Work out the finished part from the listing and answer in its coordinate system (mm). A direction names the side the tool comes from. Coordinates: 2 decimals unless noted, no trailing zeros. Write each loop counter-clockwise with the first axis right and the second up, starting at its lowest first coordinate (ties: lowest second). Pieces come first, ordered by that corner, then holes. Notation, with made-up numbers: M -39,10 L 19,10 A7 cw 19,18 Z; hole C 14,11.25 d2. An arc over 180 degrees is marked long. Use CSV: the item, a comma, the result in double quotes.
from build123d import *

# Parameters (mm, degrees)
CUT_EXTRUDE1_DEPTH      = 126.267501457
CUT_EXTRUDE1_DEPTH_BACK = 126.267501457
SKETCH2_R               = 2.986936388
CUT_EXTRUDE2_DEPTH      = 126.267501556
CUT_EXTRUDE2_DEPTH_BACK = 126.267501556


with BuildPart() as part:
    # Sketch1 → Revolve1 (revolve)
    with BuildSketch(Plane(origin=(0, 0, 0), x_dir=(0, 0, -1), z_dir=(1, 0, 0)), mode=Mode.PRIVATE) as revolve1_sk:
        Polygon((0, 123.60144971), (12, 123.60144971), (12, 86.261621461), (14.398412253, 86.261621461), (14.398412253, 79.261621461), (6.991481123, 79.261621461), (6.991481123, 8.748152398), (13.363236745, 8.748152398), (13.363236745, 3.47746721), (0, 3.47746721), align=None)
    revolve(revolve1_sk.sketch.rotate(Axis((0, 123.60144971, 0), (0, -1, 0)), 180), axis=Axis((0, 123.60144971, 0), (0, -1, 0)))

    # Sketch2 → Cut-Extrude1 (cut, two sides: drawn at the far end of the back side and taken through both)
    with BuildSketch(Plane(origin=(0, 0, 0), x_dir=(0, 0, -1), z_dir=(1, 0, 0)).offset(-CUT_EXTRUDE1_DEPTH_BACK)):
        with Locations((0, 113.066011559)):
            Circle(SKETCH2_R)
    extrude(amount=CUT_EXTRUDE1_DEPTH + CUT_EXTRUDE1_DEPTH_BACK, mode=Mode.SUBTRACT)

    # Sketch3 → Cut-Extrude2 (cut, two sides: drawn at the far end of the back side and taken through both)
    with BuildSketch(Plane(origin=(0, 0, 0), x_dir=(0, 0, -1), z_dir=(1, 0, 0)).offset(-CUT_EXTRUDE2_DEPTH_BACK)):
        with BuildLine():
            Line((1.8, 55.325549997), (1.8, 35.81578841))
            ThreePointArc((1.8, 35.81578841), (0, 34.01578841), (-1.8, 35.81578841))
            Line((-1.8, 35.81578841), (-1.8, 55.325549997))
            ThreePointArc((-1.8, 55.325549997), (0, 57.125549997), (1.8, 55.325549997))
        make_face()
    extrude(amount=CUT_EXTRUDE2_DEPTH + CUT_EXTRUDE2_DEPTH_BACK, mode=Mode.SUBTRACT)


solid = part.part
Item 1: Given pin 1 (4 mm diameter, centred on y = 91.5, z = 0.5, fed in from -X); pin 2 (4 mm diameter, centred on y = 107.5, z = -10.5, fed in from +X); pin 3 (15 mm diameter, centred on x = -3, y = 45.5, fed in from -Z), each flat-ended and moving along its own axis, determine where each tip first touches the part or whether it passes through.
Answer:
pin 1,"stops at x = -12"
pin 2,"stops at x = 8.47"
pin 3,"stops at z = -6.99"
Item 2: The part is cut by section C-C (y = 85). Write down the section's boundary in (x, z), then the cut area to 3 significant figures.
Answer:
outline,"C 0,0 d28.8"
area,"651 mm2"
Item 3: The part is cut by section A-A (z = 0). Write down the section's boundary in (x, y), then the cut area to 3 significant figures.
Answer:
outline,"M -14.4,79.26 L -6.99,79.26 L -6.99,57.13 L 6.99,57.13 L 6.99,79.26 L 14.4,79.26 L 14.4,86.26 L 12,86.26 L 12,110.08 L -12,110.08 L -12,86.26 L -14.4,86.26 Z; M -13.36,3.48 L 13.36,3.48 L 13.36,8.75 L 6.99,8.75 L 6.99,34.02 L -6.99,34.02 L -6.99,8.75 L -13.36,8.75 Z; M -12,116.05 L 12,116.05 L 12,123.6 L -12,123.6 Z"
area,"1,760 mm2"
Item 4: The part is cut by section D-D (z = -4.5). Write down the section's boundary in (x, y), then the cut area to 3 significant figures.
Answer:
outline,"M -13.68,79.26 L -5.35,79.26 L -5.35,8.75 L -12.58,8.75 L -12.58,3.48 L 12.58,3.48 L 12.58,8.75 L 5.35,8.75 L 5.35,79.26 L 13.68,79.26 L 13.68,86.26 L 11.12,86.26 L 11.12,123.6 L -11.12,123.6 L -11.12,86.26 L -13.68,86.26 Z"
area,"1,910 mm2"
Item 5: Consider probe 1 along Y at (x, z) = (6.75, 0); probe 2 along Y at (x, z) = (-2.75, 11.25); probe 3 along Y at (x, z) = (-1, 12). Determine where each line is inside the solid, lowest interval first.
Answer:
probe 1,"y = 3.48 to 34.02, 57.13 to 110.08, 116.05 to 123.6"
probe 2,"y = 3.48 to 8.75, 79.26 to 123.6"
probe 3,"y = 3.48 to 8.75, 79.26 to 86.26"
Item 6: A tool of negligible diameter and unlimited length cuts with its end or side. For faces 1 (the face through (8.761, 82.713, -11.426)), 2 (the face through (0, 46, -1.8)), 3 (the face through (4.596, 104.67, 11.085)), 4 (the face through (6, 8.748, -6)), 5 (the face through (-0.59, 6.08, -13.35)), from which of +Z, -Z, +X, -X, +Y, -Y can it reach the whole face along a straight path? Write none if from no direction.
Answer:
face 1,"+Y, -Y"
face 2,"+X, -X"
face 3,"+Y"
face 4,"none"
face 5,"-Y"
Item 7: The part is cut by section B-B (x = 0). Write down the section's boundary in (y, z), then the cut area to 3 significant figures.
Answer:
outline,"M 3.48,-13.36 L 8.75,-13.36 L 8.75,-6.99 L 79.26,-6.99 L 79.26,-14.4 L 86.26,-14.4 L 86.26,-12 L 123.6,-12 L 123.6,12 L 86.26,12 L 86.26,14.4 L 79.26,14.4 L 79.26,6.99 L 8.75,6.99 L 8.75,13.36 L 3.48,13.36 Z; hole M 35.82,-1.8 L 55.33,-1.8 A1.8 ccw 55.33,1.8 L 35.82,1.8 A1.8 ccw Z; hole C 113.07,0 d5.97"
area,"2,120 mm2"
Item 8: For a pull along Y with two mould halves and no side action, classify faces 6 (the face through (0, 3.477, 0)), 7 (the face through (-12, 86.262, 3)), 8 (the face through (-0.098, 34.016, -0.04)) as released by +Y, released by -Y, zero draft, split by the parting line, or undercut.
Answer:
face 6,"released by -Y"
face 7,"released by +Y"
face 8,"undercut"
